from build123d import *

# Parameters (mm, degrees)
SKETCH1_R           = 5
BOSS_EXTRUDE1_DEPTH = 5
FILLET2_R           = 1


with BuildPart() as part:
    # Sketch1 → Boss-Extrude1 (new body)
    with BuildSketch(Plane(origin=(0, 0, 0), x_dir=(0, 0, -1), z_dir=(1, 0, 0))):
        with BuildLine():
            Line((3.834545484, -9.235597487), (15.508521108, -4.767007874))
            ThreePointArc((15.508521108, -4.767007874), (19, 0), (15.508521108, 4.767007874))
            Line((15.508521108, 4.767007874), (3.834545484, 9.235597487))
            ThreePointArc((3.834545484, 9.235597487), (-10, 0), (3.834545484, -9.235597487))
        make_face()
        Circle(SKETCH1_R, mode=Mode.SUBTRACT)
    extrude(amount=BOSS_EXTRUDE1_DEPTH)

    # Fillet2
    # the kernel refuses this fillet: 1 mm, written as the material it adds along each edge
    with BuildSketch(Plane(origin=(0, -9.235597487, -3.834545484), x_dir=(0, -0.3828536121528857, 0.9238090233708955), z_dir=(1, 0, 0))) as fillet2_piece_1:
        with BuildLine():
            CenterArc((0.013662307, 0.999999788), FILLET2_R, 268.43540008, 1.527324084)
            Line((-0.01364172, 0.000372613), (0, 0))
            ThreePointArc((0, 0), (0.00650586, 2.116e-06), (0.013011721, 0))
        make_face()
    extrude(amount=5)
    with BuildSketch(Plane(origin=(0, 9.235597487, -3.834545484), x_dir=(0, -0.35748716903167743, -0.9339180499260719), z_dir=(1, 0, 0))) as fillet2_piece_2:
        with BuildLine():
            CenterArc((0.013646808, 1), FILLET2_R, 268.472675916, 1.527324084)
            ThreePointArc((-0.013006869, 0.000355272), (-0.006503377, 0.000179752), (0, 0))
            Line((0, 0), (0.013646808, 0))
        make_face()
    extrude(amount=5)
    with BuildSketch(Plane(origin=(0, 4.767007874, -15.508521108), x_dir=(0, 0.3574871690316874, 0.9339180499260681), z_dir=(1, 0, 0))) as fillet2_piece_3:
        with BuildLine():
            CenterArc((0.028209357, -1), FILLET2_R, 90, 3.090872231)
            ThreePointArc((-0.025710379, -0.001454727), (-0.012854253, -0.000743916), (0, 0))
            Line((0, 0), (0.028209357, 0))
        make_face()
    extrude(amount=5)
    with BuildSketch(Plane(origin=(0, -4.767007874, -15.508521108), x_dir=(0, -0.3574871690316535, 0.933918049926081), z_dir=(1, 0, 0))) as fillet2_piece_4:
        with BuildLine():
            CenterArc((0.028209357, 1), FILLET2_R, 266.909127769, 3.090872231)
            ThreePointArc((-0.025710379, 0.001454727), (-0.012854253, 0.000743916), (0, 0))
            Line((0, 0), (0.028209357, 0))
        make_face()
    extrude(amount=5)
    # the kernel refuses this fillet: 1 mm, written as the material it takes off along each edge
    with BuildSketch(Plane(origin=(5, 0, -14), x_dir=(0, -0.9518350677637516, -0.3066105082595415), z_dir=(0, -0.3066105082595415, 0.9518350677637516))) as fillet2_2_piece_1:
        with BuildLine():
            CenterArc((5 - FILLET2_R, -FILLET2_R), FILLET2_R, 0, 90)
            Line((5, -FILLET2_R), (5, 0))
            Line((5, 0), (5 - FILLET2_R, 0))
        make_face()
    revolve(axis=Axis((5, 0, -14), (1, 0, 0)), revolution_arc=144.289835586, mode=Mode.SUBTRACT)
    with BuildSketch(Plane(origin=(5, 4.777092357, -15.482175881), x_dir=(-1, 0, 0), z_dir=(0, 0.3574871690316615, 0.933918049926078)), Plane(origin=(0, -9.230718928, -3.847290484), x_dir=(0, 0.9339180499260781, 0.35748716903166156), z_dir=(0, 0.3574871690316615, -0.933918049926078))) as fillet2_2_piece_2:
        with BuildLine():
            CenterArc((FILLET2_R, FILLET2_R), FILLET2_R, 180, 90)
            Line((0, FILLET2_R), (0, 0))
            Line((0, 0), (FILLET2_R, 0))
        make_face()
    extrude(amount=12.458143836, mode=Mode.SUBTRACT)
    with BuildSketch(Plane(origin=(5, 0, 0), x_dir=(0, 0.9240579070749063, -0.38225251388623166), z_dir=(0, -0.38225251388623166, -0.9240579070749063))) as fillet2_2_piece_3:
        with BuildLine():
            CenterArc((10 - FILLET2_R, -FILLET2_R), FILLET2_R, 0, 90)
            Line((10, -FILLET2_R), (10, 0))
            Line((10, 0), (10 - FILLET2_R, 0))
        make_face()
    revolve(axis=Axis((5, 0, 0), (1, 0, 0)), revolution_arc=224.946557044, mode=Mode.SUBTRACT)
    with BuildSketch(Plane(origin=(5, -9.230718928, -3.847290484), x_dir=(0, 0.9339180499260781, 0.35748716903166156), z_dir=(0, 0.3574871690316615, -0.933918049926078)), Plane(origin=(0, 4.777092357, -15.482175881), x_dir=(1, 0, 0), z_dir=(0, 0.3574871690316615, 0.933918049926078))) as fillet2_2_piece_4:
        with BuildLine():
            CenterArc((FILLET2_R, -FILLET2_R), FILLET2_R, 90, 90)
            Line((0, -FILLET2_R), (0, 0))
            Line((0, 0), (FILLET2_R, 0))
        make_face()
    extrude(amount=12.458143836, mode=Mode.SUBTRACT)
    with BuildSketch(Plane(origin=(0, 0, 0), x_dir=(0, 0.9240579070749063, -0.38225251388623166), z_dir=(0, -0.38225251388623166, -0.9240579070749063))) as fillet2_2_piece_5:
        with BuildLine():
            CenterArc((10 - FILLET2_R, FILLET2_R), FILLET2_R, 270, 90)
            Line((10, FILLET2_R), (10, 0))
            Line((10, 0), (10 - FILLET2_R, 0))
        make_face()
    revolve(axis=Axis((0, 0, 0), (1, 0, 0)), revolution_arc=224.946557044, mode=Mode.SUBTRACT)
    with BuildSketch(Plane(origin=(0, 0, -14), x_dir=(0, -0.9518350677637516, -0.3066105082595415), z_dir=(0, -0.3066105082595415, 0.9518350677637516))) as fillet2_2_piece_6:
        with BuildLine():
            CenterArc((5 - FILLET2_R, FILLET2_R), FILLET2_R, 270, 90)
            Line((5, FILLET2_R), (5, 0))
            Line((5, 0), (5 - FILLET2_R, 0))
        make_face()
    revolve(axis=Axis((0, 0, -14), (1, 0, 0)), revolution_arc=144.289835586, mode=Mode.SUBTRACT)
    with BuildSketch(Plane(origin=(0, -10.164636978, -4.204777653), x_dir=(0, 0.9240579070749084, 0.38225251388622655), z_dir=(0, -0.38225251388622655, 0.9240579070749084))) as fillet2_2_piece_7:
        with BuildLine():
            CenterArc((1 + FILLET2_R, -FILLET2_R), FILLET2_R, 90, 90)
            Line((1, -FILLET2_R), (1, 0))
            Line((1, 0), (1 + FILLET2_R, 0))
        make_face()
    revolve(axis=Axis((0, -10.164636978, -4.204777653), (-1, 0, 0)), revolution_arc=1.527324084, mode=Mode.SUBTRACT)
    with BuildSketch(Plane(origin=(0, -5.711010407, -15.83966305), x_dir=(0, 0.9339180499260777, 0.35748716903166233), z_dir=(0, -0.35748716903166233, 0.9339180499260777))) as fillet2_2_piece_8:
        with BuildLine():
            CenterArc((1 + FILLET2_R, -FILLET2_R), FILLET2_R, 90, 90)
            Line((1, -FILLET2_R), (1, 0))
            Line((1, 0), (1 + FILLET2_R, 0))
        make_face()
    revolve(axis=Axis((0, -5.711010407, -15.83966305), (-1, 0, 0)), revolution_arc=3.090872231, mode=Mode.SUBTRACT)
    with BuildSketch(Plane(origin=(0, 5.711010407, -15.83966305), x_dir=(0, -0.9339180499260777, 0.35748716903166233), z_dir=(0, 0.35748716903166233, 0.9339180499260777))) as fillet2_2_piece_9:
        with BuildLine():
            CenterArc((1 + FILLET2_R, FILLET2_R), FILLET2_R, 180, 90)
            Line((1, FILLET2_R), (1, 0))
            Line((1, 0), (1 + FILLET2_R, 0))
        make_face()
    revolve(axis=Axis((0, 5.711010407, -15.83966305), (1, 0, 0)), revolution_arc=3.090872231, mode=Mode.SUBTRACT)
    with BuildSketch(Plane(origin=(0, 10.164636978, -4.204777653), x_dir=(0, -0.9339180499260781, 0.35748716903166156), z_dir=(0, -0.35748716903166156, -0.9339180499260781))) as fillet2_2_piece_10:
        with BuildLine():
            CenterArc((1 + FILLET2_R, -FILLET2_R), FILLET2_R, 90, 90)
            Line((1, -FILLET2_R), (1, 0))
            Line((1, 0), (1 + FILLET2_R, 0))
        make_face()
    revolve(axis=Axis((0, 10.164636978, -4.204777653), (-1, 0, 0)), revolution_arc=1.527324084, mode=Mode.SUBTRACT)
    with BuildSketch(Plane(origin=(5, -10.164636978, -4.204777653), x_dir=(0, 0.9240579070749084, 0.38225251388622655), z_dir=(0, -0.38225251388622655, 0.9240579070749084))) as fillet2_2_piece_11:
        with BuildLine():
            CenterArc((1 + FILLET2_R, FILLET2_R), FILLET2_R, 180, 90)
            Line((1, FILLET2_R), (1, 0))
            Line((1, 0), (1 + FILLET2_R, 0))
        make_face()
    revolve(axis=Axis((5, -10.164636978, -4.204777653), (-1, 0, 0)), revolution_arc=1.527324084, mode=Mode.SUBTRACT)
    with BuildSketch(Plane(origin=(5, -5.711010407, -15.83966305), x_dir=(0, 0.9339180499260777, 0.35748716903166233), z_dir=(0, -0.35748716903166233, 0.9339180499260777))) as fillet2_2_piece_12:
        with BuildLine():
            CenterArc((1 + FILLET2_R, FILLET2_R), FILLET2_R, 180, 90)
            Line((1, FILLET2_R), (1, 0))
            Line((1, 0), (1 + FILLET2_R, 0))
        make_face()
    revolve(axis=Axis((5, -5.711010407, -15.83966305), (-1, 0, 0)), revolution_arc=3.090872231, mode=Mode.SUBTRACT)
    with BuildSketch(Plane(origin=(5, 10.164636978, -4.204777653), x_dir=(0, -0.9339180499260781, 0.35748716903166156), z_dir=(0, -0.35748716903166156, -0.9339180499260781))) as fillet2_2_piece_13:
        with BuildLine():
            CenterArc((1 + FILLET2_R, FILLET2_R), FILLET2_R, 180, 90)
            Line((1 + FILLET2_R, 0), (1, 0))
            Line((1, 0), (1, FILLET2_R))
        make_face()
    revolve(axis=Axis((5, 10.164636978, -4.204777653), (-1, 0, 0)), revolution_arc=1.527324084, mode=Mode.SUBTRACT)
    with BuildSketch(Plane(origin=(5, 5.711010407, -15.83966305), x_dir=(0, -0.9339180499260777, 0.35748716903166233), z_dir=(0, 0.35748716903166233, 0.9339180499260777))) as fillet2_2_piece_14:
        with BuildLine():
            CenterArc((1 + FILLET2_R, -FILLET2_R), FILLET2_R, 90, 90)
            Line((1, -FILLET2_R), (1, 0))
            Line((1, 0), (1 + FILLET2_R, 0))
        make_face()
    revolve(axis=Axis((5, 5.711010407, -15.83966305), (1, 0, 0)), revolution_arc=3.090872231, mode=Mode.SUBTRACT)


solid = part.part
Design review of the part built by this model. Coordinates are the model's own, in mm. Coordinates: 2 decimals unless noted, no trailing zeros. Order: outer loops, then holes, each group sorted by start corner. A loop starts at its lowest first (then second) coordinate and runs counter-clockwise, first axis right, second up. Notation, with made-up numbers: (13, -38.75) -> (19, -38.75) arc R26 cw to (19, -12.75) -> close; hole circle Ø2 at (-18, 21). An arc over 180 degrees is marked (long way). Use one line per item in the form item = value. Start each with the question number.
(1) Add section A-A on z = 0. State the section outline as (x, y) points, plus the area to 3 significant figures.
(2) For probe 1 along Y at (x, z) = (1.8, 0); probe 2 along Z at (x, y) = (1.2, -4.5); probe 3 along Z at (x, y) = (0.45, 1.25), list the stretches that pass through material, from the lowest coordinate up.
(3) The part is to be moulded in two halves that separate along Y. For faces 1 (the flat face through (0, -2, -5)), 2 (the cylindrical face through (4.715, -6.754, -9.476)), 3 (the cylindrical face through (2.46, -4.88, 1.08)), 4 (the cylindrical face through (2, 0, -19)), say which applies: +Y half, -Y half, draft (parallel to the pull), parting line (faces both ways), or undercut.
(4) Insertion check: pin 1 (1.5 mm diameter, centred on y = -7, z = -10, fed in from -X); pin 2 (2 mm diameter, centred on x = 3, y = 5.5, fed in from -Z). Each pin has a flat end and moves straight along its axis. Give the tip position at first contact, or say it passes through.
Answer block:
q1.outline = (0, -9) arc R1 ccw to (1, -10) -> (4, -10) arc R1 ccw to (5, -9) -> (5, -5) -> (0, -5) -> close; (0, 5) -> (5, 5) -> (5, 9) arc R1 ccw to (4, 10) -> (1, 10) arc R1 ccw to (0, 9) -> close
q1.area = 49.1 mm²
q2.probe_1 = -10 to -5, 5 to 10
q2.probe_2 = -16.18 to -2.18, 2.18 to 8.93
q2.probe_3 = -18.67 to -4.84, 4.84 to 9.76
q3.face_1 = draft
q3.face_2 = -Y half
q3.face_3 = undercut
q3.face_4 = parting line
q4.pin_1 = 0.07
q4.pin_2 = -16.18
